Could you check a few things on this drawing? It's one solid part, dimensions in mm from its lowest x, y, z. A direction names the side the tool comes from. Give positions to 0.01 mm unless a question says otherwise; leave off trailing zeros. Order: outer loops, then holes, each group sorted by start corner. A loop starts at its lowest first (then second) coordinate and runs counter-clockwise, first axis right, second up. Notation, with made-up numbers: M 44,51 L 78,51 A28 cw 78,80 Z; hole C 45,-1 d9. An arc over 180 degrees is marked long. One line per item, written item: value. Start each with the question number.
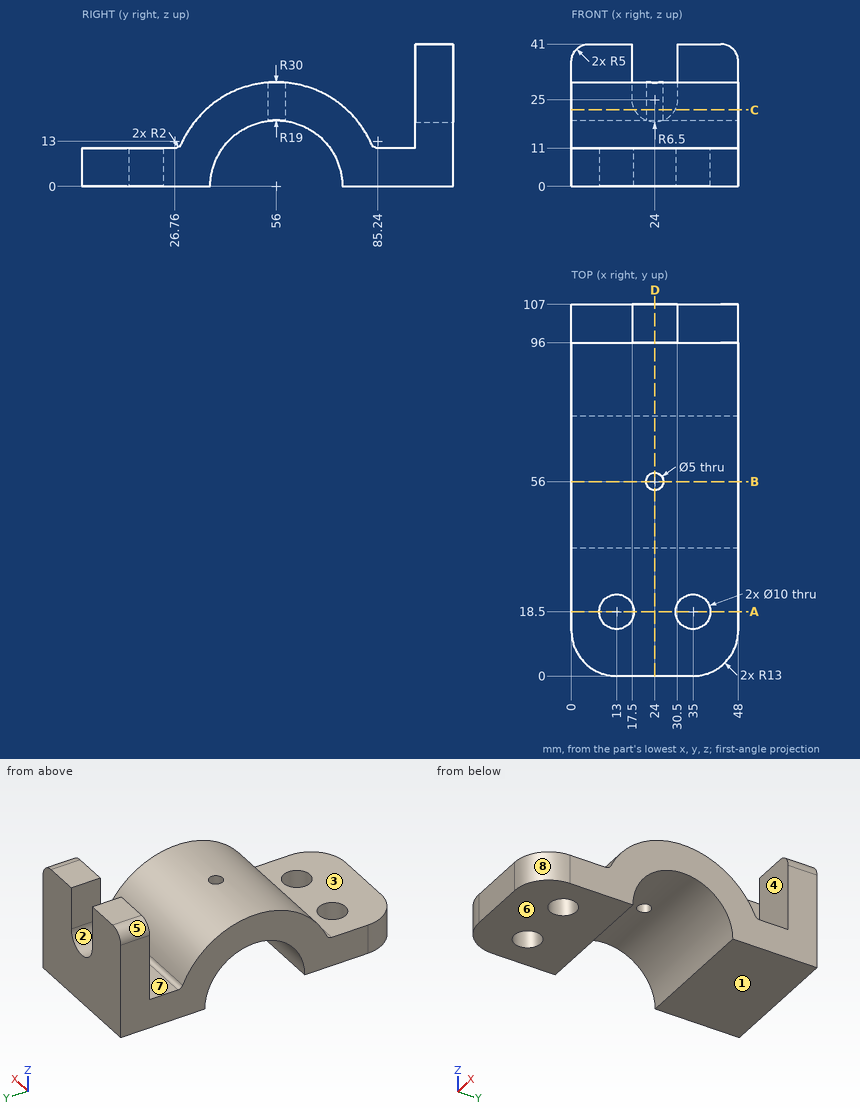
Item 1: Will these pins go through, and if not, where does the flat tip stop? P1, Ø13, axis at x = 35, y = 18.5, coming from the +Z side; P2, Ø12, axis at x = 30, y = 90.5, coming from the +Z side; P3, Ø24, axis at x = 18.5, z = 26, coming from the -Y side; P4, Ø8, axis at x = 42, y = 79, coming from the +Z side.
Item 2: I want a section at C-C on z = 22. Write out the boundary of the cut face in (x, y).
Item 3: I want a section at B-B on y = 56. Write out the boundary of the cut face in (x, z), plus the area to 3 significant figures.
Item 4: Please list where these lines run through material, in increasing order: probe 1 along X at (y, z) = (18.5, 5.25); probe 2 along X at (y, z) = (56, 25.25); probe 3 along Y at (x, z) = (16, 38). Write a range as [from, to].
Item 5: For the marked faces 1, 2, 3, 4 and 5, which set-ups out of +Z, -Z, +X, -X, +Y, -Y let a thin tool reach every point of the face, with its end or its side?
Item 6: I want a section at A-A on y = 18.5. Write out the boundary of the cut face in (x, z), plus the area to 3 significant figures.
Item 7: We'd pull the mould along Y, two halves only. Please class the marked faces 6, 7 and 8: +Y half, -Y half, draft (parallel to the pull), parting line (faces both ways), or undercut.
Item 8: I want a section at D-D on x = 24. Write out the boundary of the cut face in (y, z) (1 decimal), plus the area to 3 significant figures.
Answer below:
1. P1: stops at z = 11
1. P2: stops at z = 41
1. P3: stops at y = 29.47
1. P4: stops at z = 23.22
2. outline: M 0,35.6 L 48,35.6 L 48,76.4 L 0,76.4 Z; M 0,96 L 18.23,96 L 18.23,107 L 0,107 Z; M 29.77,96 L 48,96 L 48,107 L 29.77,107 Z; hole C 24,56 d5
3. outline: M 0,19 L 21.5,19 L 21.5,30 L 0,30 Z; M 26.5,19 L 48,19 L 48,30 L 26.5,30 Z
3. area: 473 mm²
4. probe 1: x = [0, 8], [18, 30], [40, 48]
4. probe 2: x = [0, 21.5], [26.5, 48]
4. probe 3: y = [96, 107]
5. face 1: -Z, +X, -X, +Y, -Y
5. face 2: +Z, +Y
5. face 3: +Z, +X, -X, -Y
5. face 4: +Z, +X, -X
5. face 5: +Z, -X, +Y, -Y
6. outline: M 0,0 L 8,0 L 8,11 L 0,11 Z; M 18,0 L 30,0 L 30,11 L 18,11 Z; M 40,0 L 48,0 L 48,11 L 40,11 Z
6. area: 308 mm²
7. face 6: draft
7. face 7: undercut
7. face 8: -Y half
8. outline: M 0,0 L 37,0 A19 cw 53.5,18.8 L 53.5,29.9 A30 ccw 28.6,12.2 A2 cw 26.8,11 L 0,11 Z; M 58.5,18.8 A19 cw 75,0 L 107,0 L 107,18.5 L 96,18.5 L 96,11 L 85.2,11 A2 cw 83.4,12.2 A30 ccw 58.5,29.9 Z
8. area: 1,410 mm²
